Can you work these out from the model? Positions are in its coordinate system, mm. Face numbers are marked on the shaded views. Round coordinates to 2 decimals unless told otherwise and drop trailing zeros. Loops run counter-clockwise (first coordinate to the right, second up) from the corner with the lowest first, then second, coordinate; pieces in that order, holes last.
(1) I want a section at A-A on z = -6. Write out the boundary of the cut face in (x, y) (3 decimals), plus the area to 3 significant figures.
(2) I want a section at B-B on x = -10. Write out the boundary of the cut face in (y, z) (3 decimals).
(3) Thinking about a two-plate mould opening in Y: for the marked faces 1, 2, 3 and 4, which applies, released by +Y, released by -Y, zero draft, split by the parting line, or undercut?
(4) Will these pins go through, and if not, where does the flat tip stop? pin 1 Ø0.5 at (x, y) = (30, -13.5) entering from +Z; pin 2 Ø3 at (x, z) = (31.12, 1.72) entering from +Y; pin 3 Ø2 at (x, y) = (-19, -14) entering from -Z.
(5) I want a section at C-C on z = 12. Write out the boundary of the cut face in (x, y), plus the area to 3 significant figures.
(6) If I drill on line 1 along Y through (x, z) = (19.5, 14); line 2 along X through (y, z) = (-13.05, -9.5) (3 decimals); line 3 along Z through (x, y) = (6, 5) (3 decimals), over which ranges is the centre line in solid material (lowest first)?
(7) I want a section at D-D on y = 10. Write out the boundary of the cut face in (x, z) (3 decimals), plus the area to 3 significant figures.
from build123d import *

# Parameters (mm, degrees)
SKETCH1_R            = 3.96875
BOSS_EXTRUDE1_DEPTH  = 15.286125003
SKETCH2_W            = 35.01875
SKETCH2_H            = 25.016000006
CUT_EXTRUDE1_DEPTH   = 40.686125003
SKETCH3_R            = 1.1303
CUT_EXTRUDE2_DEPTH   = 52.042953466
FILLET1_R            = 3.175
SKETCH9_R            = 1.1303
CUT_EXTRUDE5_DEPTH   = 52.042953466
FILLET1_OF_MIRROR3_R = 3.175
SKETCH7_R            = 1.4732
CUT_EXTRUDE3_DEPTH   = 55.741808709
SKETCH8_R            = 1.984375
CUT_EXTRUDE4_DEPTH   = 1.27


with BuildPart() as part:
    # Sketch1 → Boss-Extrude1 (new, symmetric)
    with BuildSketch(Plane(origin=(0, 0, 0), x_dir=(1, 0, 0), z_dir=(0, 1, 0))):
        with BuildLine():
            Line((0, -3.175), (0, -19.05))
            Line((0, -19.05), (19.05, -19.05))
            Line((19.05, -19.05), (27.573163108, -4.51))
            Line((27.573163108, -4.51), (33.923163108, -4.51))
            Line((33.923163108, -4.51), (36.048366078, 11.032185755))
            ThreePointArc((36.048366078, 11.032185755), (29.455504341, 19.1272655), (21.826728, 12))
            Line((21.826728, 12), (15.175, 12))
            Line((15.175, 12), (0, -3.175))
        make_face()
        with Locations(Location((28.970478, 12, 0), (0, 0, 270))):
            Circle(SKETCH1_R, mode=Mode.SUBTRACT)
    boss_extrude1 = extrude(amount=BOSS_EXTRUDE1_DEPTH, both=True)

    # Sketch2 → Cut-Extrude1 (cut, symmetric)
    with BuildSketch(Plane(origin=(0, 0, 0), x_dir=(0, 0, -1), z_dir=(1, 0, 0))):
        with Locations((1.634375, 0)):
            Rectangle(SKETCH2_W, SKETCH2_H)
    cut_extrude1 = extrude(amount=CUT_EXTRUDE1_DEPTH, both=True, mode=Mode.SUBTRACT)

    # Sketch3 → Cut-Extrude2 (cut, through all)
    with BuildSketch(Plane(origin=(0, 15.286125003, 0), x_dir=(1, 0, 0), z_dir=(0, 1, 0))):
        with Locations(Location((31.117871418, -1.723399824, 0), (0, 0, 270))):
            Circle(SKETCH3_R)
    cut_extrude2 = extrude(amount=-CUT_EXTRUDE2_DEPTH, mode=Mode.SUBTRACT)

    # Fillet1
    fillet1_edges = [part.edges().sort_by_distance(p)[0] for p in [
        (33.923163108, 13.897062503, 4.51),
        (27.573163108, 13.897062503, 4.51),
        (33.923163108, -13.897062503, 4.51),
        (27.573163108, -13.897062503, 4.51),
    ]]
    fillet(fillet1_edges, radius=FILLET1_R)

    # Sketch9 → Cut-Extrude5 (cut, through all)
    with BuildSketch(Plane.XZ.offset(15.286125003)):
        with Locations(Location((16.210478, -9.5, 0), (0, 0, 270))):
            Circle(SKETCH9_R)
    cut_extrude5 = extrude(amount=-CUT_EXTRUDE5_DEPTH, mode=Mode.SUBTRACT)

    # Mirror3: Boss-Extrude1, Cut-Extrude1, Cut-Extrude2, Cut-Extrude5 across plane
    add(boss_extrude1.mirror(Plane(origin=(0, 15.286125003, 3.175), x_dir=(0, 0, 1), z_dir=(1, 0, 0))))
    add(cut_extrude1.mirror(Plane(origin=(0, 15.286125003, 3.175), x_dir=(0, 0, 1), z_dir=(1, 0, 0))), mode=Mode.SUBTRACT)
    add(cut_extrude2.mirror(Plane(origin=(0, 15.286125003, 3.175), x_dir=(0, 0, 1), z_dir=(1, 0, 0))), mode=Mode.SUBTRACT)
    add(cut_extrude5.mirror(Plane(origin=(0, 15.286125003, 3.175), x_dir=(0, 0, 1), z_dir=(1, 0, 0))), mode=Mode.SUBTRACT)

    # Fillet1 of Mirror3
    fillet1_of_mirror3_edges = [part.edges().sort_by_distance(p)[0] for p in [
        (-33.923163108, 13.897062503, 4.51),
        (-27.573163108, 13.897062503, 4.51),
        (-33.923163108, -13.897062503, 4.51),
        (-27.573163108, -13.897062503, 4.51),
    ]]
    fillet(fillet1_of_mirror3_edges, radius=FILLET1_OF_MIRROR3_R)

    # Sketch7 → Cut-Extrude3 (cut, through all)
    with BuildSketch(Plane.XY.offset(19.05)):
        with Locations((-7.778174593, 7.778174593)):
            Circle(SKETCH7_R)
        with Locations((7.778174593, 7.778174593)):
            Circle(SKETCH7_R)
        with Locations((7.778174593, -7.778174593)):
            Circle(SKETCH7_R)
        with Locations((-7.778174593, -7.778174593)):
            Circle(SKETCH7_R)
    extrude(amount=-CUT_EXTRUDE3_DEPTH, mode=Mode.SUBTRACT)

    # Sketch8 → Cut-Extrude4 (cut)
    with BuildSketch(Plane(origin=(0, 15.286125003, 0), x_dir=(1, 0, 0), z_dir=(0, 1, 0))):
        with Locations(Location((31.117871418, -1.723399824, 0), (0, 0, 270))):
            Circle(SKETCH8_R)
        with Locations(Location((-31.117871418, -1.723399824, 0), (0, 0, 270))):
            Circle(SKETCH8_R)
    extrude(amount=-CUT_EXTRUDE4_DEPTH, mode=Mode.SUBTRACT)


solid = part.part
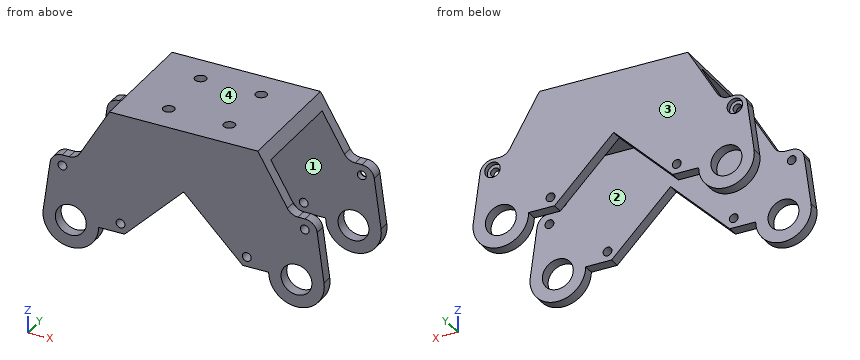
Filled sheet:
1. outline: (-35.36, -15.286) - (-9.175, -15.286) - (-9.175, -12.508) - (-35.36, -12.508) - close; (-35.36, 12.508) - (-9.175, 12.508) - (-9.175, 15.286) - (-35.36, 15.286) - close; (9.175, -15.286) - (35.36, -15.286) - (35.36, -12.508) - (9.175, -12.508) - close; (9.175, 12.508) - (35.36, 12.508) - (35.36, 15.286) - (9.175, 15.286) - close
1. area: 291 mm2
2. outline: (-15.286, -6.825) - (-12.508, -6.825) - (-12.508, 15.875) - (12.508, 15.875) - (12.508, -6.825) - (15.286, -6.825) - (15.286, 19.05) - (-15.286, 19.05) - close
3. face 1: undercut
3. face 2: undercut
3. face 3: released by +Y
3. face 4: zero draft
4. pin 1: stops at z = 4.51
4. pin 2: stops at y = 14.02
4. pin 3: stops at z = -12
5. outline: (-23.18, -15.29) - (23.18, -15.29) - (23.18, -12.51) - (-23.18, -12.51) - close; (-23.18, 12.51) - (23.18, 12.51) - (23.18, 15.29) - (-23.18, 15.29) - close
5. area: 258 mm2
6. line 1: y = -15.29 to -12.51, 12.51 to 15.29
6. line 2: x = -35.839 to -32.053, -25.888 to -17.341, -15.08 to -12.675, 12.675 to 15.08, 17.341 to 25.888, 32.053 to 35.839
6. line 3: z = 15.875 to 19.05
7. outline: (-20.911, 15.875) - (20.911, 15.875) - (19.05, 19.05) - (-19.05, 19.05) - close
7. area: 127 mm2
